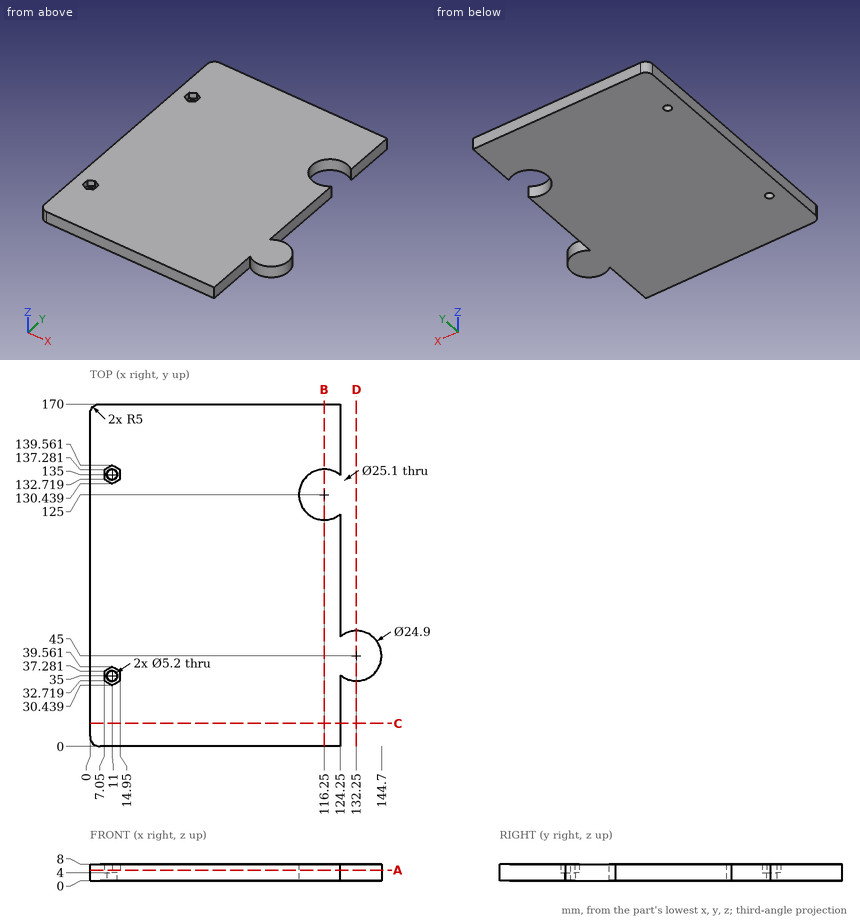
Study the drawing (mm; zero at the part's minimum x, y, z) and answer. Round coordinates to 2 decimals unless told otherwise and drop trailing zeros. Write each loop counter-clockwise with the first axis right and the second up, starting at its lowest first coordinate (ties: lowest second). Pieces come first, ordered by that corner, then holes.
1) A cutting plane is placed at D-D (x = 132.25). Give the vertices of the cut face in (y, z), plus the area to 3 significant figures.
2) Straight lines are drawn through the part: line 1 (Y direction, x = 11, z = 2.35); line 2 (Y direction, x = 116.25, z = 3); line 3 (X direction, y = 93.5, z = 7.5). For each, find the intervals that lie inside material, in ascending order.
3) A cutting plane is placed at C-C (y = 11.5). Give the vertices of the cut face in (x, z).
4) A cutting plane is placed at A-A (z = 5.25). Give the vertices of the cut face in (x, y), plus the area to 3 significant figures.
5) A cutting plane is placed at B-B (x = 116.25). Give the vertices of the cut face in (y, z).
6) Given pin 1 Ø4 at (x, y) = (11, 35) entering from -Z; pin 2 Ø2 at (y, z) = (34.5, 6.5) entering from +X (1 decimal); pin 3 Ø6 at (x, y) = (11, 135) entering from +Z; pin 4 Ø1.2 at (y, z) = (135, 6.5) entering from +X, each flat-ended and moving along its own axis, determine where each tip first touches the part or whether it passes through.
Completed:
1. outline: (32.55, 0) - (57.45, 0) - (57.45, 8) - (32.55, 8) - close
1. area: 199 mm2
2. line 1: y = 0 to 32.4, 37.6 to 132.4, 137.6 to 170
2. line 2: y = 0 to 112.45, 137.55 to 170
2. line 3: x = 0 to 124.25
3. outline: (0, 0) - (124.25, 0) - (124.25, 8) - (0, 8) - close
4. outline: (0, 5) arc R5 ccw to (5, 0) - (124.25, 0) - (124.25, 35.46) arc R12.45 ccw (long way) to (124.25, 54.54) - (124.25, 115.33) arc R12.55 cw (long way) to (124.25, 134.67) - (124.25, 170) - (5, 170) arc R5 ccw to (0, 165) - close; hole (7.05, 32.72) - (11, 30.44) - (14.95, 32.72) - (14.95, 37.28) - (11, 39.56) - (7.05, 37.28) - close; hole (7.05, 132.72) - (11, 130.44) - (14.95, 132.72) - (14.95, 137.28) - (11, 139.56) - (7.05, 137.28) - close
4. area: 21,000 mm2
5. outline: (0, 0) - (112.45, 0) - (112.45, 8) - (0, 8) - close; (137.55, 0) - (170, 0) - (170, 8) - (137.55, 8) - close
6. pin 1: passes through
6. pin 2: stops at x = 140.3
6. pin 3: stops at z = 4
6. pin 4: stops at x = 124.25
